Can you work these out from the model? Positions are in its coordinate system, mm. A direction names the side the tool comes from. Give positions to 0.01 mm unless a question says otherwise; leave off trailing zeros. Order: outer loops, then holes, each group sorted by start corner. A loop starts at its lowest first (then second) coordinate and runs counter-clockwise, first axis right, second up. Notation, with made-up numbers: M 89,-32.75 L 144,-32.75 A15 ccw 144,-9.75 Z; hole C 29,66 d6. An arc over 180 degrees is marked long. Use one line per item in the form item = value. Start each with the question number.
1. For faces 1 (the face through (0, 2, 1.5)), 2 (the face through (0, 0, -1.5)), 3 (the face through (-5.3, -6.9, 0)), which set-ups out of +Z, -Z, +X, -X, +Y, -Y let a thin tool reach every point of the face, with its end or its side?
2. I need wall thicknesses on L1, parallel to X at y = -11.2, z = 10.5; L2, parallel to Z at x = 14.65, y = -11.95; L3, parallel to Y at x = -2, z = 0. Which ranges of each line are inside material? Lowest first, please.
3. I want a section at C-C, the plane x = 4. List the corners of the cut face in (y, z) for me.
4. We'd pull the mould along X, two halves only. Please class faces 4 (the face through (24.65, -3, 1)), 5 (the face through (-24.65, -3, 1)), 6 (the face through (0, -9.65, 9)), 7 (the face through (5.3, -6.8, 0)): +X half, -X half, draft (parallel to the pull), parting line (faces both ways), or undercut.
5. I want a section at D-D, the plane y = -6.85. List the corners of the cut face in (x, z) for me.
6. I want a section at B-B, the plane y = 0.5. List the corners of the cut face in (x, z) for me (3 decimals).
7. Will these pins go through, and if not, where does the flat tip stop? P1, Ø10, axis at x = 9, y = -2.5, coming from the -Z side; P2, Ø7.5, axis at x = -7, z = 7.5, coming from the +Y side; P3, Ø3, axis at x = 7.5, y = -5.5, coming from the +Z side.
8. I want a section at A-A, the plane z = 10.5. List the corners of the cut face in (x, y) for me.
```python
from build123d import *

# Parameters (mm, degrees)
SKETCH1_W                                           = 49.3
SKETCH1_H                                           = 25.3
BOSS_EXTRUDE1_DEPTH                                 = 1.5
SKETCH4_W                                           = 49.3
SKETCH4_H                                           = 3
BOSS_EXTRUDE2_DEPTH                                 = 15
CSK_FOR_M2_COUNTERSUNK_FLAT_HEAD_SCREW1_D           = 2.4
CSK_FOR_M2_COUNTERSUNK_FLAT_HEAD_SCREW1_CSINK_D     = 4.4
CSK_FOR_M2_COUNTERSUNK_FLAT_HEAD_SCREW1_CSINK_ANGLE = 90
CUT_EXTRUDE1_REACH                                  = 33.506
SKETCH8_R                                           = 8.075


with BuildPart() as part:
    # Sketch1 → Boss-Extrude1 (new, symmetric)
    with BuildSketch(Plane.XY):
        Rectangle(SKETCH1_W, SKETCH1_H)
    extrude(amount=BOSS_EXTRUDE1_DEPTH, both=True)

    # Sketch4 → Boss-Extrude2 (add)
    with BuildSketch(Plane.XY.offset(1.5)):
        with Locations((0, -11.15)):
            Rectangle(SKETCH4_W, SKETCH4_H)
    extrude(amount=BOSS_EXTRUDE2_DEPTH)

    # CSK for M2 Countersunk Flat Head Screw1 (through all)
    with Locations(Plane(origin=(0, -9.65, 0), x_dir=(1, 0, 0), z_dir=(0, 1, 0))):
        with Locations((-14.65, -10.5), (14.65, -10.5)):
            CounterSinkHole(CSK_FOR_M2_COUNTERSUNK_FLAT_HEAD_SCREW1_D / 2, CSK_FOR_M2_COUNTERSUNK_FLAT_HEAD_SCREW1_CSINK_D / 2, counter_sink_angle=CSK_FOR_M2_COUNTERSUNK_FLAT_HEAD_SCREW1_CSINK_ANGLE)

    # Sketch8 → Cut-Extrude1 (cut, up to next)
    with BuildSketch(Plane.XY.offset(1.5), mode=Mode.PRIVATE) as cut_extrude1_sk1:
        with Locations((-13.25, 0.5)):
            Circle(SKETCH8_R)
    cut_extrude1_tool1 = extrude(cut_extrude1_sk1.sketch, amount=-CUT_EXTRUDE1_REACH, mode=Mode.PRIVATE) & part.part
    # Sketch8 → Cut-Extrude1 (cut, up to next)
    with BuildSketch(Plane.XY.offset(1.5), mode=Mode.PRIVATE) as cut_extrude1_sk2:
        with Locations((13.25, 0.5)):
            Circle(SKETCH8_R)
    cut_extrude1_tool2 = extrude(cut_extrude1_sk2.sketch, amount=-CUT_EXTRUDE1_REACH, mode=Mode.PRIVATE) & part.part
    # Sketch8 → Cut-Extrude1 (cut, up to next)
    with BuildSketch(Plane.XY.offset(1.5), mode=Mode.PRIVATE) as cut_extrude1_sk3:
        with BuildLine():
            Line((-3.3, -4.85), (3.3, -4.85))
            ThreePointArc((3.3, -4.85), (5.3, -6.85), (3.3, -8.85))
            Line((3.3, -8.85), (-3.3, -8.85))
            ThreePointArc((-3.3, -8.85), (-5.3, -6.85), (-3.3, -4.85))
        make_face()
    cut_extrude1_tool3 = extrude(cut_extrude1_sk3.sketch, amount=-CUT_EXTRUDE1_REACH, mode=Mode.PRIVATE) & part.part
    add(cut_extrude1_tool1.solids().sort_by_distance((-13.25, 0.5, 1.5))[0], mode=Mode.SUBTRACT)
    add(cut_extrude1_tool2.solids().sort_by_distance((13.25, 0.5, 1.5))[0], mode=Mode.SUBTRACT)
    add(cut_extrude1_tool3.solids().sort_by_distance((0, -6.85, 1.5))[0], mode=Mode.SUBTRACT)


solid = part.part
```
Check result:
q1.face_1 = +Z, +X, -X, +Y
q1.face_2 = -Z, +X, -X, +Y, -Y
q1.face_3 = +Z, -Z
q2.L1 = -24.65 to -15.85, -13.45 to 13.45, 15.85 to 24.65
q2.L2 = -1.5 to 9.3, 11.7 to 16.5
q2.L3 = -12.65 to -8.85, -4.85 to 12.65
q3.outline = M -12.65,-1.5 L -8.72,-1.5 L -8.72,1.5 L -9.65,1.5 L -9.65,16.5 L -12.65,16.5 Z; M -4.98,-1.5 L 12.65,-1.5 L 12.65,1.5 L -4.98,1.5 Z
q4.face_4 = +X half
q4.face_5 = -X half
q4.face_6 = draft
q4.face_7 = undercut
q5.outline = M -24.65,-1.5 L -16.59,-1.5 L -16.59,1.5 L -24.65,1.5 Z; M -9.91,-1.5 L -5.3,-1.5 L -5.3,1.5 L -9.91,1.5 Z; M 5.3,-1.5 L 9.91,-1.5 L 9.91,1.5 L 5.3,1.5 Z; M 16.59,-1.5 L 24.65,-1.5 L 24.65,1.5 L 16.59,1.5 Z
q6.outline = M -24.65,-1.5 L -21.325,-1.5 L -21.325,1.5 L -24.65,1.5 Z; M -5.175,-1.5 L 5.175,-1.5 L 5.175,1.5 L -5.175,1.5 Z; M 21.325,-1.5 L 24.65,-1.5 L 24.65,1.5 L 21.325,1.5 Z
q7.P1 = -1.5
q7.P2 = -9.65
q7.P3 = 1.5
q8.outline = M -24.65,-12.65 L -15.85,-12.65 L -15.85,-10.65 L -16.85,-9.65 L -24.65,-9.65 Z; M -13.45,-12.65 L 13.45,-12.65 L 13.45,-10.65 L 12.45,-9.65 L -12.45,-9.65 L -13.45,-10.65 Z; M 15.85,-12.65 L 24.65,-12.65 L 24.65,-9.65 L 16.85,-9.65 L 15.85,-10.65 Z
